Can you work these out from the model? Positions are in its coordinate system, mm. Coordinates: 2 decimals unless noted, no trailing zeros. Loops run counter-clockwise (first coordinate to the right, second up) from the corner with the lowest first, then second, coordinate; pieces in that order, holes last.
Autodesk Inventor part; units mm, degrees
ref_plane "YZ Plane" through (0, 0, 0) normal (1, 0, 0) x (0, 1, 0)
ref_plane "XZ Plane" through (0, 0, 0) normal (0, 1, 0) x (-1, 0, 0)
ref_plane "XY Plane" through (0, 0, 0) normal (0, 0, 1) x (1, 0, 0)
sketch "Sketch1" plane through (0, 0, 0) normal (0, 0, 1) x (1, 0, 0)
  line L0 (-71.9595, -8.3565) -> (72.0387, -7.6433)
  line L1 (72.0387, -7.6433) -> (71.7812, 44.356)
  line L2 (71.7812, 44.356) -> (49.7815, 44.2471)
  line L3 (49.7815, 44.2471) -> (49.9598, 8.2475)
  line L4 (49.9598, 8.2475) -> (-46.0391, 7.7721)
  line L5 (-46.0391, 7.7721) -> (-46.2173, 43.7717)
  line L6 (-46.2173, 43.7717) -> (-56.2172, 43.7221)
  line L7 (-71.9595, -8.3565) -> (-71.9595, 27.7497)
  line L8 (-71.9595, 27.7497) -> (-56.2172, 43.7221)
  point P0 (0, 0)
  dimension "d0" = 144
  dimension "d1" = 52
  dimension "d2" = 22
  dimension "d3" = 36
  dimension "d4" = 96
  dimension "d5" = 36
  dimension "d6" = 10
  dimension "d8" = 72
  dimension "d9" = 16
  dimension "d10" = 8
extrude "Extrusion1" add sketch "Sketch1" along normal blind 64
sketch "Sketch3" plane through (71.7812, 44.356, 64) normal (0.9999877, 0.0049523, 0) x (0, 0, -1)
  line L0 (64, -52) -> (64, 0)
  line L1 (0, -52) -> (0, 0)
  line L2 (48, -52) -> (48, -45)
  line L3 (40, -45) -> (40, -36)
  line L4 (48, -45) -> (40, -45)
  line L5 (40, -36) -> (32, -36)
  line L6 (64, -36) -> (0, -36)
  line L7 (16, -52) -> (16, -45)
  line L8 (24, -45) -> (24, -36)
  line L9 (16, -45) -> (24, -45)
  line L10 (24, -36) -> (32, -36)
  line L11 (16, -52) -> (48, -52)
  line L12 (64, -52) -> (0, -52)
  line L13 (64, -36) -> (64, 0)
  arc A0 (58.5136, -26.6786) -> (61, -28) centre (61, -25) ccw
  arc A1 (45.2611, -7.0477) -> (18.7389, -7.0477) centre (32, -16) ccw
  circle A2 centre (32, -16) radius 8
  line L14 (64, 0) -> (0, 0)
  line L15 (45.2611, -7.0477) -> (58.5136, -26.6786)
  line L16 (64, -28) -> (61, -28)
  line L17 (64, -15.8943) -> (0, -15.8943)
  arc A3 (3, -28) -> (5.4864, -26.6786) centre (3, -25) ccw
  line L18 (18.7389, -7.0477) -> (5.4864, -26.6786)
  line L19 (0, -28) -> (3, -28)
  line L20 (0, -36) -> (0, 0)
  line L21 (0, -28) -> (0, 0)
  line L22 (64, 0) -> (0, 0)
  line L23 (0, 0) -> (64, 0)
  line L24 (64, 0) -> (64, -28)
  point P0 (64, -44)
  point P1 (32, 0)
  point P2 (0, -28)
  point P3 (64, -28)
  dimension "d13" = 64
  dimension "d16" = 7
  dimension "d18" = 32
  dimension "d19" = 16
  dimension "d20" = 16
  dimension "d21" = 9
  dimension "d24" = 24
  dimension "d26" = 6
  dimension "d27" = 32
  dimension "d28" = 16
  dimension "d29" = 32
  dimension "d30" = 64
extrude "Extrusion2" cut sketch "Sketch3" against normal through all contours L11 L7 L9 L8 L6 L5 L3 L4 L2
extrude "Extrusion3" cut sketch "Sketch3" against normal blind 22 contours L16 A0 L15 L17 L0 | L17 L15 A1 L14 L0 | A1 L18 L17 L1 L14 | L17 A2 | A2 L17 | L1 L17 L18 A3 L19
sketch "Sketch4" plane through (-45.9598, -8.2277, 64) normal (-0.0049523, 0.9999877, 0) x (0.9999877, 0.0049523, 0)
  line L0 (118, 16) -> (118, 0)
  line L1 (96, 0) -> (0, 0)
  circle A0 centre (80, 10) radius 3
  circle A1 centre (10, 10) radius 3
  line L2 (-40.7838, 32) -> (143.3901, 32)
  circle A2 centre (80, 54) radius 3
  circle A3 centre (10, 54) radius 3
  point P0 (46, 64)
  dimension "d35" = 6
  dimension "d37" = 6
extrude "Extrusion4" cut sketch "Sketch4" along normal blind 15
equation "\"d29\" = 0.5 * d30"
properties part number "Parte2_Base" material "Steel, Carbon"
Item 1: Suppose I cut it at B-B, the plane z = 26. Please give me the cut outline in (x, y), plus the area to 3 significant figures.
Results are:
outline: (-71.96, 7.64) - (-46.04, 7.77) - (-46.22, 43.77) - (-56.22, 43.72) - (-71.96, 27.75) - close; (49.79, 43.08) - (49.83, 33.54) - (71.83, 33.65) - (71.79, 43.19) - close; (49.89, 22.96) - (49.96, 8.25) - (71.96, 8.36) - (71.89, 23.06) - close
area: 1,340 mm2
Item 2: Suppose I cut it at C-C, the plane y = 2. Count the separate pieces of the cut face and the enclosed holes in it, plus the area to 3 significant figures.
Results are:
separate pieces: 2
enclosed holes: 4
area: 6,800 mm2
Item 3: Suppose I cut it at A-A, the plane x = 43.5. Please give me the cut outline in (y, z).
Results are:
outline: (-7.78, 0) - (8.22, 0) - (8.22, 24) - (-0.78, 24) - (-0.78, 16) - (-7.78, 16) - close; (-7.78, 48) - (-0.78, 48) - (-0.78, 40) - (8.22, 40) - (8.22, 64) - (-7.78, 64) - close
Item 4: I'm going to push flat-ended pins straight in: P1, Ø5, axis at x = -51.5, z = 39.5, coming from the +Y side; P2, Ø1.5, axis at x = 51, z = 16, coming from the +Y side; P3, Ø1, axis at y = 5, z = 22, coming from the +X side; P4, Ø10.5, axis at x = 30, y = 2, coming from the -Z side. Where does each tip first touch, or does it pass through?
Results are:
P1: stops at y = 43.76
P2: stops at y = 34.26
P3: stops at x = 71.98
P4: stops at z = 0
Item 5: We'd pull the mould along Z, two halves only. Please class faces 1 (the face through (-17, 6, 64)), 2 (the face through (-36, -1, 57)), 3 (the face through (-33.225, -0.769, 8.851)), 4 (the face through (-71.96, 13, 32)): +Z half, -Z half, draft (parallel to the pull), parting line (faces both ways), or undercut.
Results are:
face 1: +Z half
face 2: undercut
face 3: undercut
face 4: draft
Item 6: I need wall thicknesses on line 1 along X through (y, z) = (12.5, 7.5); line 2 along Z through (x, y) = (14, 8); line 3 along X through (y, z) = (10, 34.5). Which ranges of each line are inside material? Lowest first, please.
Results are:
line 1: x = -71.96 to -46.06, 49.94 to 71.94
line 2: z = 0 to 24, 40 to 64
line 3: x = -71.96 to -46.05, 49.95 to 71.95
Item 7: Suppose I cut it at D-D, the plane z = 36.5. Please give me the cut outline in (x, y).
Results are:
outline: (-71.96, 7.64) - (-46.04, 7.77) - (-46.22, 43.77) - (-56.22, 43.72) - (-71.96, 27.75) - close; (49.78, 43.6) - (49.83, 34.86) - (71.83, 34.97) - (71.78, 43.71) - close; (49.89, 21.63) - (49.96, 8.25) - (71.96, 8.36) - (71.89, 21.74) - close
